Source: CAD feature listing. Evaluate the final solid. Frame: model axes, mm. Face numbers are marked on the shaded views. A direction names the side the tool comes from. Give positions to 0.01 mm unless a question says otherwise; leave off trailing zeros. Order: outer loops, then holes, each group sorted by start corner. A loop starts at its lowest first (then second) coordinate and runs counter-clockwise, first axis right, second up. Notation, with made-up numbers: M 53.25,70.25 L 110.25,70.25 A18 ccw 110.25,95.25 Z; hole C 11,21.5 d7. An arc over 180 degrees is marked long. Use CSV: the item, a comma, the result in double quotes. Start each with the question number.
Item 1: First-contact query: pin 1 (4 mm diameter, centred on x = -41, z = 14.5, fed in from +Y); pin 2 (16 mm diameter, centred on y = 6, z = 24, fed in from -X); pin 3 (10 mm diameter, centred on y = 7.5, z = 29, fed in from +X). Flat tips, straight axial feed; report the tip coordinate or a pass-through.
Item 2: Access query for the marked faces 1, 2 and 3. Directions: +Z, -Z, +X, -X, +Y, -Y. A direction counts if a zero-diameter tool reaches every point of the face in a straight line with its end or side. Return the directions, or none.
Item 3: Ray query, probe 1 along Z at (x, y) = (0, 22.1); probe 2 along Y at (x, z) = (8.5, 8); probe 3 along X at (y, z) = (-8, 24). Return the intervals inside material, ascending. Write a range as from..to.
Item 4: Section query C-C on y = -51. Return loops of the section in (x, z), and give its area (3 significant figures).
Item 5: Pull-direction query (X, two-part tool) for the marked faces 4, 5 and 6; classes: +X half, -X half, draft (parallel to the pull), parting line (faces both ways), or undercut.
Item 6: Section query B-B on z = 20. Return loops of the section in (x, y) (3 decimals).
Item 7: Section query D-D on z = 37. Return loops of the section in (x, y) (3 decimals).
Item 8: Section query A-A on x = 0. Return loops of the section in (y, z), and give its area (3 significant figures).
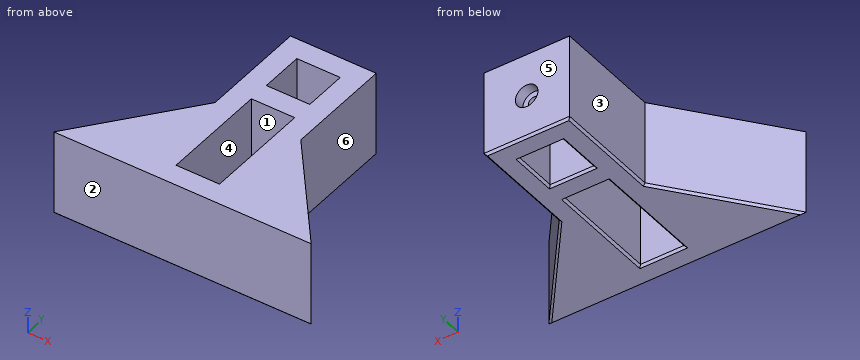
from build123d import *

# Parameters (mm, degrees)
SKETCH1_W           = 20.25
SKETCH1_H           = 20.25
SKETCH1_H_2         = 50
BOSS_EXTRUDE1_DEPTH = 40
CHAMFER1_SIZE       = 1
SKETCH2_R           = 2.75
CUT_EXTRUDE1_DEPTH  = 20
SKETCH3_R           = 5.25
CUT_EXTRUDE2_DEPTH  = 5


with BuildPart() as part:
    # Sketch1 → Boss-Extrude1 (new body)
    with BuildSketch(Plane.XY):
        Polygon((20, -19.875), (60, -70), (20, -70), (-20, -70), (-60, -70), (-20, -19.875), (-20, 30.25), (20, 30.25), align=None)
        with Locations((0.125, 10.125)):
            Rectangle(SKETCH1_W, SKETCH1_H, mode=Mode.SUBTRACT)
        with Locations((0.125, -35)):
            Rectangle(SKETCH1_W, SKETCH1_H_2, mode=Mode.SUBTRACT)
    extrude(amount=BOSS_EXTRUDE1_DEPTH)

    # Chamfer1
    chamfer1_edges = [part.edges().sort_by_distance(p)[0] for p in [
        (-40, -44.9375, 0),
        (-20, 5.1875, 0),
        (-10, 10.125, 0),
        (0.125, 0, 0),
        (10.25, 10.125, 0),
        (0.125, 20.25, 0),
        (-10, -35, 0),
        (0.125, -60, 0),
        (10.25, -35, 0),
        (0.125, -10, 0),
        (0, 30.25, 0),
        (20, 5.1875, 0),
        (40, -44.9375, 0),
        (0, -70, 0),
    ]]
    chamfer(chamfer1_edges, length=CHAMFER1_SIZE)

    # Sketch2 → Cut-Extrude1 (cut)
    with BuildSketch(Plane(origin=(0, 30.25, 0), x_dir=(1, 0, 0), z_dir=(0, 1, 0))):
        with Locations(Location((0, -20, 0), (0, 0, 180))):
            Circle(SKETCH2_R)
    extrude(amount=-CUT_EXTRUDE1_DEPTH, mode=Mode.SUBTRACT)

    # Sketch3 → Cut-Extrude2 (cut)
    with BuildSketch(Plane(origin=(0, 30.25, 0), x_dir=(1, 0, 0), z_dir=(0, 1, 0))):
        with Locations(Location((0, -20, 0), (0, 0, 180))):
            Circle(SKETCH3_R)
    extrude(amount=-CUT_EXTRUDE2_DEPTH, mode=Mode.SUBTRACT)


solid = part.part
Verdict:
1,pin 1,"y = -43.68"
1,pin 2,"x = -20"
1,pin 3,"x = 20"
2,face 1,"+Z, -Z"
2,face 2,"+Z, -Z, +X, -X, -Y"
2,face 3,"+Z, -Z, -X, +Y"
3,probe 1,"0..17.25, 22.75..40"
3,probe 2,"-70..-60, -10..0, 20.25..30.25"
3,probe 3,"-20..20"
4,outline,"M -44.84,1 L -43.56,0 L -11,0 L -10,1 L -10,40 L -44.84,40 Z; M 10.25,1 L 11.25,0 L 43.56,0 L 44.84,1 L 44.84,40 L 10.25,40 Z"
4,area,"2,770 mm2"
5,face 4,"undercut"
5,face 5,"draft"
5,face 6,"+X half"
6,outline,"M -60,-70 L 60,-70 L 20,-19.875 L 20,30.25 L 5.25,30.25 L 5.25,25.25 L 2.75,25.25 L 2.75,20.25 L 10.25,20.25 L 10.25,0 L -10,0 L -10,20.25 L -2.75,20.25 L -2.75,25.25 L -5.25,25.25 L -5.25,30.25 L -20,30.25 L -20,-19.875 Z; hole M -10,-60 L 10.25,-60 L 10.25,-10 L -10,-10 Z"
7,outline,"M -60,-70 L 60,-70 L 20,-19.875 L 20,30.25 L -20,30.25 L -20,-19.875 Z; hole M -10,-60 L 10.25,-60 L 10.25,-10 L -10,-10 Z; hole M -10,0 L 10.25,0 L 10.25,20.25 L -10,20.25 Z"
8,outline,"M -70,1 L -69,0 L -61,0 L -60,1 L -60,40 L -70,40 Z; M -10,1 L -9,0 L -1,0 L 0,1 L 0,40 L -10,40 Z; M 20.25,1 L 21.25,0 L 29.25,0 L 30.25,1 L 30.25,14.75 L 25.25,14.75 L 25.25,17.25 L 20.25,17.25 Z; M 20.25,22.75 L 25.25,22.75 L 25.25,25.25 L 30.25,25.25 L 30.25,40 L 20.25,40 Z"
8,area,"1,120 mm2"
